Part model, mm, in its own coordinate system. A direction names the side the tool comes from. Coordinates: 2 decimals unless noted, no trailing zeros. Answer as a JSON object with one key per item and string values. Group by question number.
1. 3-axis set-ups, long thin cutter, end or side, ignore diameter. For faces 1 (the face through (2, 2.675, -12.2)), 2 (the face through (13.277, 2.502, -2.948)), 3 (the face through (-6, -1.955, -9)), 4 (the face through (7.079, -1.475, -8.392)), 5 (the face through (-11.5, -0.105, 5.3)): which of +Z, -Z, +X, -X, +Y, -Y reach the whole face in a straight line?
2. Drill centre lines: L1, parallel to Y at x = -5.5, z = 11.5 (3 decimals); L2, parallel to X at y = -1.15, z = -7.5; L3, parallel to X at y = -1.7, z = 3. Where is each one in solid material? Low to high.
3. Mould opens along Z. For faces 6 (the face through (-7.106, -1.475, -8.425)), 7 (the face through (0, -2.675, 0)), 8 (the face through (5.362, 1.127, 12.932)) say: released by +Z, released by -Z, zero draft, split by the parting line, or undercut.
4. Drop flat-ended pins along their axis: pin 1 Ø3 at (x, y) = (-2, -1) entering from -Z; pin 2 Ø10 at (x, z) = (-1.5, 0.5) entering from +Y; pin 3 Ø2 at (x, y) = (9.5, 0.5) entering from -Z. Give the stop position or say it passes through.
from build123d import *
from build123d.topology import SkipClean

# Parameters (mm, degrees)
BOSS_EXTRUDE1_DEPTH = 0.75
SKETCH4_RX          = 1.303717269
SKETCH4_RY          = 0.905346041
BOSS_EXTRUDE2_DEPTH = 0.1
FILLET1_R           = 0.1


with BuildPart() as part:
    # Sketch1 → Revolve1 (revolve)
    with BuildSketch(Plane(origin=(0, 0, 0), x_dir=(0, 0, -1), z_dir=(1, 0, 0)), mode=Mode.PRIVATE) as revolve1_sk:
        Polygon((0, 2.675), (0, -2.675), (6.65, -2.675), (6.65, -1.105), (12.5, -1.105), (12.5, -0.105), (14, -0.105), (14, 2.325), (13.6, 2.325), (13.6, 2.675), align=None)
    revolve(revolve1_sk.sketch.rotate(Axis((0, 2.675, 0), (0, -1, 0)), 180), axis=Axis((0, 2.675, 0), (0, -1, 0)))

    # Sketch2 → Cut-Revolve1 (revolve, cut)
    with BuildSketch(Plane.XY):
        with BuildLine():
            Line((12.167843198, 2.675), (12.167843198, 4.188369308))
            Line((12.167843198, 4.188369308), (0, 4.188369308))
            Line((0, 4.188369308), (0, 2.20930679))
            add(Edge.make_bspline(
                [(0, 2.20930679), (0.697493383, 2.096114571), (1.712976925, 2.479358765), (3.089812768, 2.524529264), (5.522613834, 1.273374007), (10.13555892, 1.104929536), (12.167843198, 2.675)],
                knots=[0, 0, 0, 0, 0.198883602, 0.334629802, 0.396962893, 1, 1, 1, 1], degree=3))
        make_face()
    revolve(axis=Axis((0, -2.675, 0), (0, 1, 0)), mode=Mode.SUBTRACT)

    # Sketch3 → Boss-Extrude1 (add)
    with SkipClean():  # the faces are left unmerged after this step: merging them gives an invalid solid
        with BuildSketch(Plane.XZ.offset(1.105)):
            with BuildLine():
                Line((6.125, -7.261843774), (8.059210526, -9.555057598))
                ThreePointArc((8.059210526, -9.555057598), (0, -12.5), (-8.059210526, -9.555057598))
                Line((-8.059210526, -9.555057598), (-6.125, -7.261843774))
                ThreePointArc((-6.125, -7.261843774), (0, -9.5), (6.125, -7.261843774))
            make_face()
        extrude(amount=BOSS_EXTRUDE1_DEPTH)

    # Sketch4 → Boss-Extrude2 (add)
    with SkipClean():  # the faces are left unmerged after this step: merging them gives an invalid solid
        with BuildSketch(Plane.XZ.offset(1.855)):
            with Locations(Location((6.168922757, -8.940301825), (0, 0, -55.097504384))):
                Ellipse(SKETCH4_RX, SKETCH4_RY)
            with Locations(Location((-6.168922757, -8.940301825), (0, 0, -124.902495616))):
                Ellipse(SKETCH4_RX, SKETCH4_RY)
        extrude(amount=BOSS_EXTRUDE2_DEPTH)

    # Fillet1
    fillet1_edges = [part.edges().sort_by_distance(p)[0] for p in [
        (5.42295973, -1.955, -7.871088152),
        (-5.42295973, -1.955, -7.871088152),
    ]]
    fillet(fillet1_edges, radius=FILLET1_R - 0.0001)  # a hair under: the kernel refuses the full size


solid = part.part
Outcome:
{
 "1": {"face 1": "+Z, -Z, +X, -X, +Y", "face 2": "+Y", "face 3": "-Z, +X, -X, -Y", "face 4": "+X, -Y", "face 5": "-Y"},
 "2": {"L1": "y = -0.105 to 2.675", "L2": "x = -6.33 to -5.83, 5.83 to 6.33", "L3": "x = -5.93 to 5.93"},
 "3": {"face 6": "undercut", "face 7": "zero draft", "face 8": "split by the parting line"},
 "4": {"pin 1": "stops at z = -13.98", "pin 2": "stops at y = 2.48", "pin 3": "stops at z = -11.12"}
}
